The model under review builds one solid part; all positions refer to its coordinate system, in mm. A direction names the side the tool comes from. Coordinates: 2 decimals unless noted, no trailing zeros. Order: outer loops, then holes, each group sorted by start corner. A loop starts at its lowest first (then second) coordinate and runs counter-clockwise, first axis right, second up.
```python
from build123d import *

# Parameters (mm, degrees)
BOSS_EXTRUDE1_DEPTH = 5
BOSS_EXTRUDE2_DEPTH = 15
CUT_EXTRUDE1_DEPTH  = 15
SKETCH4_W           = 2
SKETCH4_H           = 2
CUT_EXTRUDE2_DEPTH  = 15


with BuildPart() as part:
    # Sketch1 → Boss-Extrude1 (new body)
    with BuildSketch(Plane.XY):
        with BuildLine():
            Line((-19.818415432, 19.704812021), (-8.818415432, 19.704812021))
            Line((-8.818415432, 19.704812021), (-8.818415432, 6.204812021))
            Line((-8.818415432, 6.204812021), (-10.318415432, 4.704812021))
            Line((-10.318415432, 4.704812021), (-11.318415432, 4.704812021))
            ThreePointArc((-11.318415432, 4.704812021), (-14.318415432, 7.704812021), (-17.318415432, 4.704812021))
            Line((-17.318415432, 4.704812021), (-18.318415432, 4.704812021))
            Line((-18.318415432, 4.704812021), (-19.818415432, 6.204812021))
            Line((-19.818415432, 6.204812021), (-19.818415432, 19.704812021))
        make_face()
    extrude(amount=BOSS_EXTRUDE1_DEPTH)

    # Sketch2 → Boss-Extrude2 (add)
    with BuildSketch(Plane(origin=(0, 19.704812021, 0), x_dir=(1, 0, 0), z_dir=(0, 1, 0))):
        Polygon((-19.818415432, -1.5), (-8.818415432, -1.5), (-7.850169596, -1.75), (-7.850169596, -3.25), (-8.818415432, -3.5), (-19.818415432, -3.5), (-20.786661269, -3.25), (-20.786661269, -1.75), align=None)
    extrude(amount=-BOSS_EXTRUDE2_DEPTH)

    # Sketch3 → Cut-Extrude1 (cut)
    with BuildSketch(Plane.XY.offset(5)):
        with BuildLine():
            Line((-18.318415432, 4.704812021), (-20.786661269, 7.173057858))
            Line((-20.786661269, 7.173057858), (-20.786661269, 3.709596772))
            Line((-20.786661269, 3.709596772), (-7.850169596, 3.709596772))
            Line((-7.850169596, 3.709596772), (-7.850169596, 7.173057858))
            Line((-7.850169596, 7.173057858), (-10.318415432, 4.704812021))
            Line((-10.318415432, 4.704812021), (-11.318415432, 4.704812021))
            ThreePointArc((-11.318415432, 4.704812021), (-14.318415432, 7.704812021), (-17.318415432, 4.704812021))
            Line((-17.318415432, 4.704812021), (-18.318415432, 4.704812021))
        make_face()
    extrude(amount=-CUT_EXTRUDE1_DEPTH, mode=Mode.SUBTRACT)

    # Sketch4 → Cut-Extrude2 (cut)
    with BuildSketch(Plane.XY.offset(5)):
        with Locations((-19.786661269, 13.704812021)):
            Rectangle(SKETCH4_W, SKETCH4_H)
    cut_extrude2 = extrude(amount=-CUT_EXTRUDE2_DEPTH, mode=Mode.SUBTRACT)

    # Mirror1: Cut-Extrude2 across plane
    add(cut_extrude2.mirror(Plane(origin=(-14.318415432, 0, 0), x_dir=(0, 0, 1), z_dir=(1, 0, 0))), mode=Mode.SUBTRACT)


solid = part.part
```
(1) We need section C-C, the plane y = 5.75. Write out the cut boundary in (x, z).
A:
outline: (-19.36, 0) - (-17.13, 0) - (-17.13, 5) - (-19.36, 5) - close; (-11.51, 0) - (-9.27, 0) - (-9.27, 5) - (-11.51, 5) - close
(2) We need section B-B, the plane z = 1. Write out the cut boundary in (x, y), and give its area (3 significant figures).
A:
outline: (-19.82, 6.2) - (-18.32, 4.7) - (-17.32, 4.7) arc R3 cw to (-11.32, 4.7) - (-10.32, 4.7) - (-8.82, 6.2) - (-8.82, 12.7) - (-9.85, 12.7) - (-9.85, 14.7) - (-8.82, 14.7) - (-8.82, 19.7) - (-19.82, 19.7) - (-19.82, 14.7) - (-18.79, 14.7) - (-18.79, 12.7) - (-19.82, 12.7) - close
area: 144 mm2
(3) Draft analysis for pull direction Y (two halves, no side actions). For faces 1 (the face through (-8.341, 9.5, 1.623)), 2 (the face through (-20, 14.705, 3)), 3 (the face through (-14.252, 7.704, 2.465)), state which applies: released by +Y, released by -Y, zero draft, split by the parting line, or undercut.
A:
face 1: zero draft
face 2: undercut
face 3: released by -Y
(4) For pin 1 Ø0.8 at (y, z) = (17.5, 4) entering from +X; pin 2 Ø1 at (x, z) = (-9, 3.5) entering from -Y; pin 3 Ø1.6 at (x, z) = (-19.5, 1.5) entering from -Y, all flat-tipped, find the tip position at first contact; note any pin that passes through.
A:
pin 1: stops at x = -8.82
pin 2: stops at y = 5.52
pin 3: stops at y = 5.09
(5) Wall thickness on probe 1 along X at (y, z) = (12, 4.85); probe 2 along X at (y, z) = (7.25, 3.2); probe 3 along X at (y, z) = (13, 4.75): over which ranges is each line inside the solid? List them lowest first.
A:
probe 1: x = -19.82 to -8.82
probe 2: x = -20.79 to -15.91, -12.73 to -7.85
probe 3: x = -18.79 to -9.85
(6) Machinability: for faces 4 (the face through (-8.818, 10, 4)), 5 (the face through (-18.787, 14, 3)), 6 (the face through (-8.818, 10, 1)), which of the approach directions +Z, -Z, +X, -X, +Y, -Y give a long, thin tool a straight path to every point of the face, cutting with its end or side? Answer none if there is none.
A:
face 4: +Z, +X, +Y, -Y
face 5: +Z, -Z, -X
face 6: -Z, +X, +Y, -Y
(7) We need section D-D, the plane x = -19.5. Write out the cut boundary in (y, z), and give its area (3 significant figures).
A:
outline: (5.89, 0) - (12.7, 0) - (12.7, 5) - (5.89, 5) - close; (14.7, 0) - (19.7, 0) - (19.7, 5) - (14.7, 5) - close
area: 59.1 mm2
(8) We need section A-A, the plane y = 8.25. Write out the cut boundary in (x, z), and give its area (3 significant figures).
A:
outline: (-20.79, 1.75) - (-19.82, 1.5) - (-19.82, 0) - (-8.82, 0) - (-8.82, 1.5) - (-7.85, 1.75) - (-7.85, 3.25) - (-8.82, 3.5) - (-8.82, 5) - (-19.82, 5) - (-19.82, 3.5) - (-20.79, 3.25) - close
area: 58.4 mm2
